Verification items for the finished model (mm, model axes). A direction names the side the tool comes from. Coordinates: 2 decimals unless noted, no trailing zeros. Loops run counter-clockwise (first coordinate to the right, second up) from the corner with the lowest first, then second, coordinate; pieces in that order, holes last. Notation, with made-up numbers: (-1, 33.5) -> (18, 33.5) arc R12 cw to (18, 41.5) -> close; hole circle Ø3 at (39, 81.25). An arc over 180 degrees is marked (long way). Use CSV: the item, a comma, the result in double quotes. Start each with the question number.
```python
from build123d import *

# Parameters (mm, degrees)
F0_R     = 31.75
F1_DEPTH = 12.7
F2_R     = 13.335
F3_DEPTH = 25.4


with BuildPart() as f1:
    # F0 (on Top) → F1 (new body)
    with BuildSketch(Plane.XY):
        Circle(F0_R)
        with BuildLine():
            ThreePointArc((-10.794772, -22.992018), (-21.997045, -12.7), (-25.309058, 2.147462))
            ThreePointArc((-25.309058, 2.147462), (-21.876993, 5.042662), (-18.981793, 1.610597))
            ThreePointArc((-18.981793, 1.610597), (-16.497784, -9.525), (-8.096079, -17.244014))
            ThreePointArc((-8.096079, -17.244014), (-6.571423, -21.467362), (-10.794772, -22.992018))
        make_face(mode=Mode.SUBTRACT)
        with BuildLine():
            ThreePointArc((25.309058, 2.147462), (21.997045, -12.7), (10.794772, -22.992018))
            ThreePointArc((10.794772, -22.992018), (6.571423, -21.467362), (8.096079, -17.244014))
            ThreePointArc((8.096079, -17.244014), (16.497784, -9.525), (18.981793, 1.610597))
            ThreePointArc((18.981793, 1.610597), (21.876993, 5.042662), (25.309058, 2.147462))
        make_face(mode=Mode.SUBTRACT)
        with BuildLine():
            ThreePointArc((10.885714, 15.633417), (0, 19.05), (-10.885714, 15.633417))
            ThreePointArc((-10.885714, 15.633417), (-15.305569, 16.424701), (-14.514286, 20.844556))
            ThreePointArc((-14.514286, 20.844556), (0, 25.4), (14.514286, 20.844556))
            ThreePointArc((14.514286, 20.844556), (15.305569, 16.424701), (10.885714, 15.633417))
        make_face(mode=Mode.SUBTRACT)
    extrude(amount=F1_DEPTH)

    # F2 (on face) → F3 (cut)
    with BuildSketch(Plane.XY.offset(12.7)):
        Circle(F2_R)
    extrude(amount=-F3_DEPTH, mode=Mode.SUBTRACT)


solid = f1.part
```
1. Set-up check for faces 1 (the cylindrical face through (-21.95, 5.05, 6.26)), 2 (the flat face through (14, 0, 0)): record each of +Z, -Z, +X, -X, +Y, -Y from which the full face is reachable in a straight line by a thin tool's end or side.
2. Depth check by flat-ended pin: pin 1 (5 mm diameter, centred on y = -4.5, z = 5, fed in from -X); pin 2 (6 mm diameter, centred on x = 2.5, z = 4.5, fed in from -Y). Enter the tip coordinate at first touch or a pass-through.
3. Cross-section at D-D, the plane y = -20. Record the boundary of the cut face in (x, z).
4. Cross-section at A-A, the plane x = 0. Record the boundary of the cut face in (y, z) (3 decimals), plus the area to 3 significant figures.
5. Cross-section at B-B, the plane y = 0. Record the boundary of the cut face in (x, z) (3 decimals), plus the area to 3 significant figures.
6. Scan lines: line 1 (X direction, y = 0.5, z = 9.5); line 2 (Y direction, x = 0, z = 8.75) (3 decimals); line 3 (X direction, y = -21, z = 0.75). Record each from-to range of solid material in increasing order.
7. Release check for a two-part mould opening along X. For faces 3 (the cylindrical face through (15.345, 16.482, 6.261)), 4 (the cylindrical face through (-6.883, -30.995, 6.261)), 5 (the flat face through (14, 0, 12.7)) record: released by +X, released by -X, zero draft, split by the parting line, or undercut.
8. Cross-section at C-C, the plane x = -17.5. Record the boundary of the cut face in (y, z).
Solution:
1,face 1,"+Z, -Z"
1,face 2,"-Z, +X, -X, +Y, -Y"
2,pin 1,"stops at x = -31.69"
2,pin 2,"stops at y = -31.75"
3,outline,"(-24.66, 0) -> (-15.66, 0) -> (-15.66, 12.7) -> (-24.66, 12.7) -> close; (-6.27, 0) -> (6.27, 0) -> (6.27, 12.7) -> (-6.27, 12.7) -> close; (15.66, 0) -> (24.66, 0) -> (24.66, 12.7) -> (15.66, 12.7) -> close"
4,outline,"(-31.75, 0) -> (-13.335, 0) -> (-13.335, 12.7) -> (-31.75, 12.7) -> close; (13.335, 0) -> (19.05, 0) -> (19.05, 12.7) -> (13.335, 12.7) -> close; (25.4, 0) -> (31.75, 0) -> (31.75, 12.7) -> (25.4, 12.7) -> close"
4,area,"387 mm2"
5,outline,"(-31.75, 0) -> (-25.4, 0) -> (-25.4, 12.7) -> (-31.75, 12.7) -> close; (-19.05, 0) -> (-13.335, 0) -> (-13.335, 12.7) -> (-19.05, 12.7) -> close; (13.335, 0) -> (19.05, 0) -> (19.05, 12.7) -> (13.335, 12.7) -> close; (25.4, 0) -> (31.75, 0) -> (31.75, 12.7) -> (25.4, 12.7) -> close"
5,area,"306 mm2"
6,line 1,"x = -31.75 to -25.4, -19.04 to -13.33, 13.33 to 19.04, 25.4 to 31.75"
6,line 2,"y = -31.75 to -13.335, 13.335 to 19.05, 25.4 to 31.75"
6,line 3,"x = -23.81 to -14.29, -6.4 to 6.4, 14.29 to 23.81"
7,face 3,"undercut"
7,face 4,"split by the parting line"
7,face 5,"zero draft"
8,outline,"(-26.49, 0) -> (-18.41, 0) -> (-18.41, 12.7) -> (-26.49, 12.7) -> close; (-7.53, 0) -> (26.49, 0) -> (26.49, 12.7) -> (-7.53, 12.7) -> close"
